Can you work these out from the model? Positions are in its coordinate system, mm. A direction names the side the tool comes from. Give positions to 0.01 mm unless a question says otherwise; leave off trailing zeros. Order: outer loops, then holes, each group sorted by start corner. A loop starts at its lowest first (then second) coordinate and runs counter-clockwise, first axis right, second up. Notation, with made-up numbers: (43, 59.5) - (68, 59.5) arc R9 ccw to (68, 71.5) - close; hole circle Ø10 at (-19.5, 37). An arc over 180 degrees is marked (long way). Return JSON: item names as keys, results as strings.
```python
from build123d import *

# Parameters (mm, degrees)
SKETCH1_W           = 330.2
SKETCH1_H           = 6.35
BOSS_EXTRUDE1_DEPTH = 25.4
BOSS_EXTRUDE2_DEPTH = 6.35
CUT_EXTRUDE1_DEPTH  = 168.16307158


with BuildPart() as part:
    # Sketch1 → Boss-Extrude1 (new body)
    with BuildSketch(Plane(origin=(0, 0, 0), x_dir=(1, 0, 0), z_dir=(0, 1, 0))):
        Rectangle(SKETCH1_W, SKETCH1_H)
    extrude(amount=BOSS_EXTRUDE1_DEPTH)

    # Sketch2 → Boss-Extrude2 (add)
    with BuildSketch(Plane.XZ):
        with BuildLine():
            Line((-133.35, 2.54), (-133.35, -2.54))
            ThreePointArc((-133.35, -2.54), (-135.89, 0), (-133.35, 2.54))
        make_face()
        with BuildLine():
            Line((-66.675, 2.54), (-66.675, -2.54))
            ThreePointArc((-66.675, -2.54), (-69.215, 0), (-66.675, 2.54))
        make_face()
        with BuildLine():
            Line((0, 2.54), (0, -2.54))
            ThreePointArc((0, -2.54), (-2.54, 0), (0, 2.54))
        make_face()
        with BuildLine():
            Line((66.675, 2.54), (66.675, -2.54))
            ThreePointArc((66.675, -2.54), (64.135, 0), (66.675, 2.54))
        make_face()
        with BuildLine():
            Line((133.35, 2.54), (133.35, -2.54))
            ThreePointArc((133.35, -2.54), (130.81, 0), (133.35, 2.54))
        make_face()
    extrude(amount=BOSS_EXTRUDE2_DEPTH)

    # Sketch3 → Cut-Extrude1 (cut, through all)
    with BuildSketch(Plane.XY.offset(3.175)):
        with BuildLine():
            Line((-143.51, 38.1), (-143.51, 12.7))
            ThreePointArc((-143.51, 12.7), (-146.05, 10.16), (-148.59, 12.7))
            Line((-148.59, 12.7), (-148.59, 38.1))
            ThreePointArc((-148.59, 38.1), (-146.05, 40.64), (-143.51, 38.1))
        make_face()
        with BuildLine():
            Line((-125.095, 38.1), (-125.095, 12.7))
            ThreePointArc((-125.095, 12.7), (-127.635, 10.16), (-130.175, 12.7))
            Line((-130.175, 12.7), (-130.175, 38.1))
            ThreePointArc((-130.175, 38.1), (-127.635, 40.64), (-125.095, 38.1))
        make_face()
        with BuildLine():
            Line((-106.68, 38.1), (-106.68, 12.7))
            ThreePointArc((-106.68, 12.7), (-109.22, 10.16), (-111.76, 12.7))
            Line((-111.76, 12.7), (-111.76, 38.1))
            ThreePointArc((-111.76, 38.1), (-109.22, 40.64), (-106.68, 38.1))
        make_face()
        with BuildLine():
            Line((-88.265, 38.1), (-88.265, 12.7))
            ThreePointArc((-88.265, 12.7), (-90.805, 10.16), (-93.345, 12.7))
            Line((-93.345, 12.7), (-93.345, 38.1))
            ThreePointArc((-93.345, 38.1), (-90.805, 40.64), (-88.265, 38.1))
        make_face()
        with BuildLine():
            Line((-69.85, 38.1), (-69.85, 12.7))
            ThreePointArc((-69.85, 12.7), (-72.39, 10.16), (-74.93, 12.7))
            Line((-74.93, 12.7), (-74.93, 38.1))
            ThreePointArc((-74.93, 38.1), (-72.39, 40.64), (-69.85, 38.1))
        make_face()
        with BuildLine():
            Line((-51.435, 38.1), (-51.435, 12.7))
            ThreePointArc((-51.435, 12.7), (-53.975, 10.16), (-56.515, 12.7))
            Line((-56.515, 12.7), (-56.515, 38.1))
            ThreePointArc((-56.515, 38.1), (-53.975, 40.64), (-51.435, 38.1))
        make_face()
        with BuildLine():
            Line((-33.02, 38.1), (-33.02, 12.7))
            ThreePointArc((-33.02, 12.7), (-35.56, 10.16), (-38.1, 12.7))
            Line((-38.1, 12.7), (-38.1, 38.1))
            ThreePointArc((-38.1, 38.1), (-35.56, 40.64), (-33.02, 38.1))
        make_face()
        with BuildLine():
            Line((-14.605, 38.1), (-14.605, 12.7))
            ThreePointArc((-14.605, 12.7), (-17.145, 10.16), (-19.685, 12.7))
            Line((-19.685, 12.7), (-19.685, 38.1))
            ThreePointArc((-19.685, 38.1), (-17.145, 40.64), (-14.605, 38.1))
        make_face()
        with BuildLine():
            Line((3.81, 38.1), (3.81, 12.7))
            ThreePointArc((3.81, 12.7), (1.27, 10.16), (-1.27, 12.7))
            Line((-1.27, 12.7), (-1.27, 38.1))
            ThreePointArc((-1.27, 38.1), (1.27, 40.64), (3.81, 38.1))
        make_face()
        with BuildLine():
            Line((22.225, 38.1), (22.225, 12.7))
            ThreePointArc((22.225, 12.7), (19.685, 10.16), (17.145, 12.7))
            Line((17.145, 12.7), (17.145, 38.1))
            ThreePointArc((17.145, 38.1), (19.685, 40.64), (22.225, 38.1))
        make_face()
        with BuildLine():
            Line((40.64, 38.1), (40.64, 12.7))
            ThreePointArc((40.64, 12.7), (38.1, 10.16), (35.56, 12.7))
            Line((35.56, 12.7), (35.56, 38.1))
            ThreePointArc((35.56, 38.1), (38.1, 40.64), (40.64, 38.1))
        make_face()
        with BuildLine():
            Line((59.055, 38.1), (59.055, 12.7))
            ThreePointArc((59.055, 12.7), (56.515, 10.16), (53.975, 12.7))
            Line((53.975, 12.7), (53.975, 38.1))
            ThreePointArc((53.975, 38.1), (56.515, 40.64), (59.055, 38.1))
        make_face()
        with BuildLine():
            Line((77.47, 38.1), (77.47, 12.7))
            ThreePointArc((77.47, 12.7), (74.93, 10.16), (72.39, 12.7))
            Line((72.39, 12.7), (72.39, 38.1))
            ThreePointArc((72.39, 38.1), (74.93, 40.64), (77.47, 38.1))
        make_face()
        with BuildLine():
            Line((95.885, 38.1), (95.885, 12.7))
            ThreePointArc((95.885, 12.7), (93.345, 10.16), (90.805, 12.7))
            Line((90.805, 12.7), (90.805, 38.1))
            ThreePointArc((90.805, 38.1), (93.345, 40.64), (95.885, 38.1))
        make_face()
        with BuildLine():
            Line((114.3, 38.1), (114.3, 12.7))
            ThreePointArc((114.3, 12.7), (111.76, 10.16), (109.22, 12.7))
            Line((109.22, 12.7), (109.22, 38.1))
            ThreePointArc((109.22, 38.1), (111.76, 40.64), (114.3, 38.1))
        make_face()
        with BuildLine():
            Line((132.715, 38.1), (132.715, 12.7))
            ThreePointArc((132.715, 12.7), (130.175, 10.16), (127.635, 12.7))
            Line((127.635, 12.7), (127.635, 38.1))
            ThreePointArc((127.635, 38.1), (130.175, 40.64), (132.715, 38.1))
        make_face()
        with BuildLine():
            Line((151.13, 38.1), (151.13, 12.7))
            ThreePointArc((151.13, 12.7), (148.59, 10.16), (146.05, 12.7))
            Line((146.05, 12.7), (146.05, 38.1))
            ThreePointArc((146.05, 38.1), (148.59, 40.64), (151.13, 38.1))
        make_face()
    extrude(amount=-CUT_EXTRUDE1_DEPTH, mode=Mode.SUBTRACT)


solid = part.part
```
1. On a 3-axis mill with a long thin cutter (end or side, diameter ignored), from which of +Z, -Z, +X, -X, +Y, -Y can I reach the whole of each face in a straight line? I mean faces 4 (the face through (10, 25.4, 0)), 5 (the face through (66.675, -3, 0)), 6 (the face through (95.885, 19, 0)). Say none if no direction works.
Checks:
{"face 4": "+Z, -Z, +X, -X, +Y", "face 5": "+Z, -Z, -Y", "face 6": "+Z, -Z, +Y"}
2. Suppose I cut it at B-B (x = -7). List the corners of the cut face in (y, z) for me (3 decimals), plus the area to 3 significant figures.
Checks:
{"outline": "(0, -3.175) - (25.4, -3.175) - (25.4, 3.175) - (0, 3.175) - close", "area": "161 mm^2"}
3. Suppose I cut it at A-A (y = 18.5). State how many separate pieces and enclosed holes the cut face has, plus the area to 3 significant figures.
Checks:
{"separate pieces": "18", "enclosed holes": "0", "area": "1,550 mm^2"}
4. Thinking about a two-plate mould opening in X: for faces 1 (the face through (-165.1, 13, 0)), 2 (the face through (102, 25.4, 0)), 3 (the face through (130.81, -3.13, -0.06)), which applies, +X half, -X half, draft (parallel to the pull), parting line (faces both ways), or undercut?
Checks:
{"face 1": "-X half", "face 2": "draft", "face 3": "undercut"}
5. For pin 1 Ø1.9 at (x, z) = (56, 0) entering from -Y; pin 2 Ø4 at (x, y) = (18, -2.5) entering from -Z; pin 3 Ø1.5 at (y, z) = (-3, 0.5) entering from +X, each with a flat end and sliding along its axis, tell me the tip position at first contact or that it passes through.
Checks:
{"pin 1": "y = 0", "pin 2": "through", "pin 3": "x = 133.35"}
6. If I drill on L1, parallel to X at y = -4.5, z = -0.25 (3 decimals); L2, parallel to X at y = -2, z = 2.25 (3 decimals); L3, parallel to Y at x = 90.5, z = 1.5, over which ranges is the centre line in solid material (lowest first)? Write a range as [from, to].
Checks:
{"L1": "[-135.878, -133.35], [-69.203, -66.675], [-2.528, 0], [64.147, 66.675], [130.822, 133.35]", "L2": "[-134.529, -133.35], [-67.854, -66.675], [-1.179, 0], [65.496, 66.675], [132.171, 133.35]", "L3": "[0, 25.4]"}
